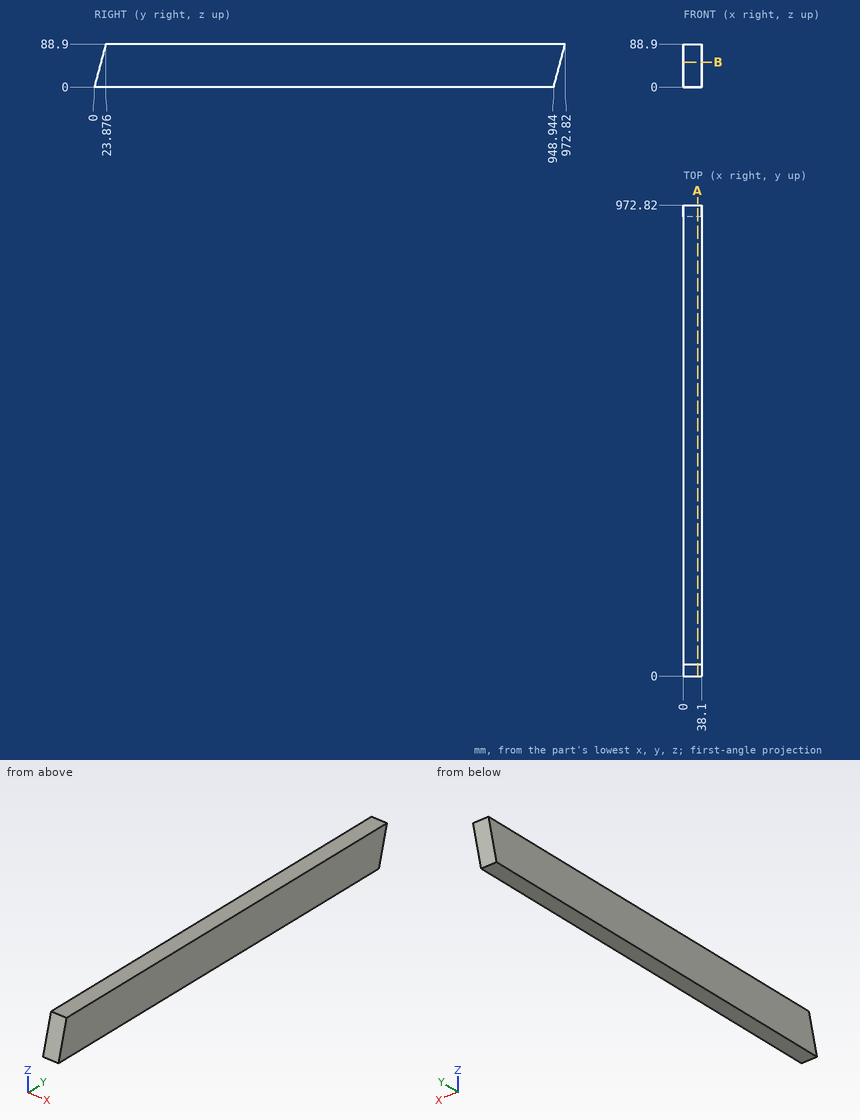
Job drawing, mm, ordinate dimensions from the low corner. One solid piece. Coordinates: 2 decimals unless noted, no trailing zeros. Order: outer loops, then holes, each group sorted by start corner. A loop starts at its lowest first (then second) coordinate and runs counter-clockwise, first axis right, second up. Notation, with made-up numbers: (-17, 51.25) - (0, 51.25) arc R19 ccw to (0, 70.25) - close; hole circle Ø6 at (13.25, 66). An arc over 180 degrees is marked (long way). Return JSON: item names as keys, results as strings. Group by question number.
1) Saw through at A-A, the plane x = 29.5. Write the cut outline in (y, z), plus the area to 3 significant figures.
2) Saw through at B-B, the plane z = 51.5. Write the cut outline in (x, y).
3) Probe line 1 (Y direction, x = 9.5, z = 65); line 2 (Y direction, x = 26, z = 80.5). List the from-to ranges inside material, lowest first. Write a range as from..to.
4) Flat gauge pin, fed straight in: P1, Ø1.5, axis at x = 31.5, z = 23, coming from the +Y side. Where does the tip first touch, or does it go through?
Values found:
{
 "1": {"outline": "(0, 0) - (948.94, 0) - (972.82, 88.9) - (23.88, 88.9) - close", "area": "84,400 mm²"},
 "2": {"outline": "(0, 13.83) - (38.1, 13.83) - (38.1, 962.78) - (0, 962.78) - close"},
 "3": {"line 1": "y = 17.46..966.4", "line 2": "y = 21.62..970.56"},
 "4": {"P1": "stops at y = 955.32"}
}
